from build123d import *

# Parameters (mm, degrees)
SKETCH1_W           = 30
SKETCH1_H           = 30
SKETCH1_R           = 1.25
BOSS_EXTRUDE2_DEPTH = 12
FILLET1_R           = 1


with BuildPart() as part:
    # Sketch1 → Boss-Extrude2 (new body)
    with BuildSketch(Plane(origin=(0, 0, 0), x_dir=(1, 0, 0), z_dir=(0, 1, 0))):
        Rectangle(SKETCH1_W, SKETCH1_H)
        with Locations((-9.25, 0)):
            Circle(SKETCH1_R, mode=Mode.SUBTRACT)
        with Locations((9.25, 0)):
            Circle(SKETCH1_R, mode=Mode.SUBTRACT)
        with Locations((0, 7.848591319)):
            Circle(SKETCH1_R, mode=Mode.SUBTRACT)
        with Locations((0, -7.651408681)):
            Circle(SKETCH1_R, mode=Mode.SUBTRACT)
        with Locations((9.300881955, 8.35126307)):
            Circle(SKETCH1_R, mode=Mode.SUBTRACT)
        with Locations((9.300881955, -9.32640646)):
            Circle(SKETCH1_R, mode=Mode.SUBTRACT)
        with Locations((-8.376787575, -9.32640646)):
            Circle(SKETCH1_R, mode=Mode.SUBTRACT)
        with Locations((-8.376787575, 8.35126307)):
            Circle(SKETCH1_R, mode=Mode.SUBTRACT)
        Polygon((4.5033321, -2.54076447), (4.5033321, 2.65923553), (0, 5.25923553), (-4.5033321, 2.65923553), (-4.5033321, -2.54076447), (0, -5.14076447), align=None, mode=Mode.SUBTRACT)
    extrude(amount=BOSS_EXTRUDE2_DEPTH)

    # Fillet1
    fillet1_edges = [part.edges().sort_by_distance(p)[0] for p in [
        (15, 6, 15),
        (-15, 6, 15),
        (-15, 6, -15),
        (15, 6, -15),
    ]]
    fillet(fillet1_edges, radius=FILLET1_R)


solid = part.part
Read the model definition and answer for the solid it produces. Units are mm, in the model's axes. A direction names the side the tool comes from. Round coordinates to 2 decimals unless told otherwise and drop trailing zeros. Write each loop counter-clockwise with the first axis right and the second up, starting at its lowest first coordinate (ties: lowest second). Pieces come first, ordered by that corner, then holes. Notation, with made-up numbers: (-9.5, 76.5) - (31.5, 76.5) arc R24 cw to (31.5, 89.5) - close; hole circle Ø7 at (1.25, -32). An arc over 180 degrees is marked (long way). Use a Markdown table: item, result.
(1) The part is cut by section A-A (z = 0). Write down the section's boundary in (x, y).
Reported:
| item | result |
|---|---|
| outline | (-15, 0) - (-10.5, 0) - (-10.5, 12) - (-15, 12) - close; (-8, 0) - (-4.5, 0) - (-4.5, 12) - (-8, 12) - close; (4.5, 0) - (8, 0) - (8, 12) - (4.5, 12) - close; (10.5, 0) - (15, 0) - (15, 12) - (10.5, 12) - close |
(2) Straight lines are drawn through the part: line 1 along Z through (x, y) = (0, 10); line 2 along X through (y, z) = (8.75, 0); line 3 along Z through (x, y) = (-9.25, 7.75). For each, find the intervals that lie inside material, in ascending order. Write a range as [from, to].
Reported:
| item | result |
|---|---|
| line 1 | [-15, -9.1], [-6.6, -5.26], [5.14, 6.4], [8.9, 15] |
| line 2 | [-15, -10.5], [-8, -4.5], [4.5, 8], [10.5, 15] |
| line 3 | [-15, -9.25], [-7.46, -1.25], [1.25, 8.43], [10.22, 15] |
(3) The part is cut by section D-D (z = -4). Write down the section's boundary in (x, y), then the cut area to 3 significant figures.
Reported:
| item | result |
|---|---|
| outline | (-15, 0) - (-2.18, 0) - (-2.18, 12) - (-15, 12) - close; (2.18, 0) - (15, 0) - (15, 12) - (2.18, 12) - close |
| area | 308 mm2 |
(4) Which of the six approach directions +Z, -Z, +X, -X, +Y, -Y give full straight-line access (tool end or side, diameter ignored) to faces 5 (the flat face through (-4.503, 6, 0)), 6 (the flat face through (-15, 6, 0))?
Reported:
| item | result |
|---|---|
| face 5 | +Y, -Y |
| face 6 | +Z, -Z, -X, +Y, -Y |
(5) The part is cut by section C-C (y = 3.25). State how many separate pieces and enclosed holes the cut face has, then the cut area to 3 significant figures.
Reported:
| item | result |
|---|---|
| separate pieces | 1 |
| enclosed holes | 9 |
| area | 790 mm2 |
(6) The mould has two halves that part along X. Classify faces 1 (the cylindrical face through (14.699, 6.084, 14.715)), 2 (the flat face through (4.503, 6, 0)), 3 (the flat face through (0, 6, -15)), 4 (the cylindrical face through (-8.54, 5.916, 8.087)): released by +X, released by -X, zero draft, split by the parting line, or undercut.
Reported:
| item | result |
|---|---|
| face 1 | released by +X |
| face 2 | undercut |
| face 3 | zero draft |
| face 4 | undercut |
(7) This flat-tipped pin is pushed along its axis until it touches: pin 1 Ø2 at (x, z) = (0, -7.85) entering from -Y. Where does it stop, or does it pass through?
Reported:
| item | result |
|---|---|
| pin 1 | through |
(8) The part is cut by section B-B (x = 9.25). Write down the section's boundary in (y, z), then the cut area to 3 significant figures.
Reported:
| item | result |
|---|---|
| outline | (0, -15) - (12, -15) - (12, -9.6) - (0, -9.6) - close; (0, -7.1) - (12, -7.1) - (12, -1.25) - (0, -1.25) - close; (0, 1.25) - (12, 1.25) - (12, 8.08) - (0, 8.08) - close; (0, 10.58) - (12, 10.58) - (12, 15) - (0, 15) - close |
| area | 270 mm2 |
